Input: part model. Units: mm. Frame: model coordinates. Face numbers are marked on the shaded views. Round coordinates to 2 decimals unless told otherwise and drop trailing zeros. Write each loop counter-clockwise with the first axis right and the second up, starting at its lowest first coordinate (ties: lowest second). Pieces come first, ordered by that corner, then holes. Notation, with made-up numbers: (69, 27.5) -> (118, 27.5) arc R27 ccw to (118, 51.5) -> close; hole circle Ø9 at (70.25, 67.5). An arc over 180 degrees is marked (long way). Use CSV: the item, a comma, the result in double quotes.
```python
from build123d import *

# Parameters (mm, degrees)
SKETCH1_W                   = 76.2
SKETCH1_H                   = 38.1
EXTRUDE1_DEPTH              = 6.35
F_1_2_CLEARANCE_HOLE1_D     = 13.89126
F_1_2_CLEARANCE_HOLE1_DEPTH = 6.35
F_1_2_CLEARANCE_HOLE1_TIP   = 4.173355541


with BuildPart() as part:
    # Sketch1 → Extrude1 (new body)
    with BuildSketch(Plane.XY):
        Rectangle(SKETCH1_W, SKETCH1_H)
    extrude(amount=-EXTRUDE1_DEPTH)

    # 1/2 Clearance Hole1
    with Locations(Plane.XY):
        with Locations((-25.4, 0), (25.4, 0)):
            Hole(F_1_2_CLEARANCE_HOLE1_D / 2, depth=F_1_2_CLEARANCE_HOLE1_DEPTH)
            with Locations((0, 0, -(F_1_2_CLEARANCE_HOLE1_DEPTH + F_1_2_CLEARANCE_HOLE1_TIP / 2))):  # 118° drill point
                Cone(0, F_1_2_CLEARANCE_HOLE1_D / 2, F_1_2_CLEARANCE_HOLE1_TIP, mode=Mode.SUBTRACT)


solid = part.part
```
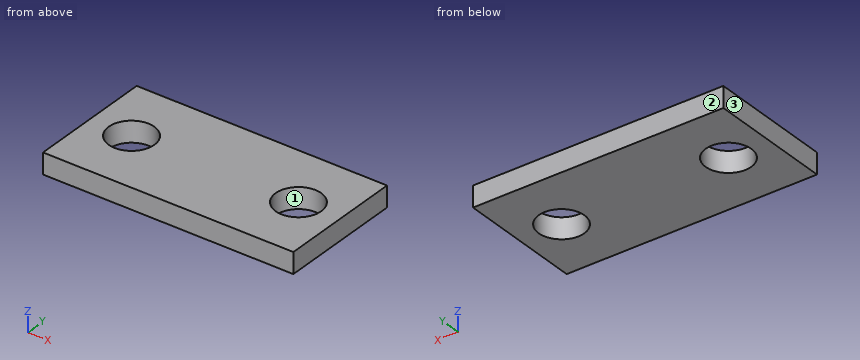
Item 1: Line query: line 1 (X direction, y = 0, z = -4.5); line 2 (Y direction, x = -25.4, z = -2.5); line 3 (Y direction, x = 23, z = -4.75). Output: solid intervals per line, ascending.
Worked answers:
line 1,"x = -38.1 to -32.35, -18.45 to 18.45, 32.35 to 38.1"
line 2,"y = -19.05 to -6.95, 6.95 to 19.05"
line 3,"y = -19.05 to -6.52, 6.52 to 19.05"
Item 2: Section query A-A on y = 0. Return the cut outline in (x, z), plus the area to 3 significant figures.
Worked answers:
outline,"(-38.1, -6.35) -> (-32.35, -6.35) -> (-32.35, 0) -> (-38.1, 0) -> close; (-18.45, -6.35) -> (18.45, -6.35) -> (18.45, 0) -> (-18.45, 0) -> close; (32.35, -6.35) -> (38.1, -6.35) -> (38.1, 0) -> (32.35, 0) -> close"
area,"307 mm²"
Item 3: Section query C-C on z = -0.75. Return the cut outline in (x, y).
Worked answers:
outline,"(-38.1, -19.05) -> (38.1, -19.05) -> (38.1, 19.05) -> (-38.1, 19.05) -> close; hole circle Ø13.89 at (-25.4, 0); hole circle Ø13.89 at (25.4, 0)"
Item 4: Pull-direction query (X, two-part tool) for the marked faces 1, 2 and 3; classes: +X half, -X half, draft (parallel to the pull), parting line (faces both ways), or undercut.
Worked answers:
face 1,"undercut"
face 2,"draft"
face 3,"-X half"
Item 5: Section query B-B on x = 25.4. Return the cut outline in (y, z).
Worked answers:
outline,"(-19.05, -6.35) -> (-6.95, -6.35) -> (-6.95, 0) -> (-19.05, 0) -> close; (6.95, -6.35) -> (19.05, -6.35) -> (19.05, 0) -> (6.95, 0) -> close"
